from build123d import *

# Parameters (mm, degrees)
SKETCH1_W               = 50
SKETCH1_H               = 79
SKETCH1_R               = 1.7
SKETCH1_W_2             = 25.4
SKETCH1_H_2             = 47.625
BOSS_EXTRUDE1_DEPTH     = 5
SKETCH2_W               = 20
SKETCH2_H               = 5
BOSS_EXTRUDE2_DEPTH     = 50
FILLET1_R               = 10
CUT_EXTRUDE1_DEPTH      = 86.240835285
CUT_EXTRUDE1_DEPTH_BACK = 86.240835285
SKETCH3_R               = 2


with BuildPart() as part:
    # Sketch1 → Boss-Extrude1 (new body)
    with BuildSketch(Plane.XY):
        Rectangle(SKETCH1_W, SKETCH1_H)
        with Locations((-20, 0)):
            Circle(SKETCH1_R, mode=Mode.SUBTRACT)
        with Locations((20, 0)):
            Circle(SKETCH1_R, mode=Mode.SUBTRACT)
        Rectangle(SKETCH1_W_2, SKETCH1_H_2, mode=Mode.SUBTRACT)
    extrude(amount=BOSS_EXTRUDE1_DEPTH)

    # Sketch2 → Boss-Extrude2 (add)
    with BuildSketch(Plane.ZY.offset(25)):
        with Locations((-10, 37)):
            Rectangle(SKETCH2_W, SKETCH2_H)
        with Locations((-10, -37)):
            Rectangle(SKETCH2_W, SKETCH2_H)
    extrude(amount=-BOSS_EXTRUDE2_DEPTH)

    # Fillet1
    fillet1_edges = [part.edges().sort_by_distance(p)[0] for p in [
        (0, 34.5, 0),
        (0, -34.5, 0),
    ]]
    fillet(fillet1_edges, radius=FILLET1_R)

    # Sketch3 → Cut-Extrude1 (cut, two sides: drawn at the far end of the back side and taken through both)
    with BuildSketch(Plane(origin=(0, 39.5, 0), x_dir=(1, 0, 0), z_dir=(0, 1, 0)).offset(-CUT_EXTRUDE1_DEPTH_BACK)):
        with Locations((-17.5, 10)):
            Circle(SKETCH3_R)
        with Locations((-6, 10)):
            Circle(SKETCH3_R)
        with Locations(Location((6, 10, 0), (0, 0, 180))):
            Circle(SKETCH3_R)
        with Locations((17.5, 10)):
            Circle(SKETCH3_R)
    extrude(amount=CUT_EXTRUDE1_DEPTH + CUT_EXTRUDE1_DEPTH_BACK, mode=Mode.SUBTRACT)


solid = part.part
Here's how the part is built. I have some questions about the finished solid (model axes, mm). A direction names the side the tool comes from. Round coordinates to 2 decimals unless told otherwise and drop trailing zeros. Order: outer loops, then holes, each group sorted by start corner. A loop starts at its lowest first (then second) coordinate and runs counter-clockwise, first axis right, second up. Notation, with made-up numbers: M 43.25,20 L 51.25,20 A4 ccw 51.25,26 Z; hole C 21.25,45 d4. An arc over 180 degrees is marked long. Return JSON: item names as keys, results as strings. Group by question number.
1. Please list where these lines run through material, in increasing order: probe 1 along Y at (x, z) = (-14, -13); probe 2 along Y at (x, z) = (20, 4); probe 3 along Z at (x, y) = (-6, -35.95).
2. I'm going to push flat-ended pins straight in: pin 1 Ø12 at (x, y) = (-15.5, -24) entering from -Z; pin 2 Ø2.5 at (x, z) = (-17.5, -10) entering from -Y; pin 3 Ø1.5 at (x, y) = (13, -23) entering from -Z. Where does each tip first touch, or does it pass through?
3. If we section it at D-D on x = -17.5: List the corners of the cut face in (y, z) for me, then the cut area to 3 significant figures.
4. On a 3-axis mill with a long thin cutter (end or side, diameter ignored), from which of +Z, -Z, +X, -X, +Y, -Y can I reach the whole of each face in a straight line? I mean faces 3 (the face through (-18.974, 36.863, -11.352)), 4 (the face through (-12.7, 0, 2)), 5 (the face through (0.35, -31.65, -3.01)). Say none if no direction works.
5. If we section it at A-A on x = 6: List the corners of the cut face in (y, z) for me, then the cut area to 3 significant figures.
6. If we section it at B-B on z = -17: List the corners of the cut face in (x, y) for me, then the cut area to 3 significant figures.
7. If we mould it in two halves opening along Y, with no side actions, what happens to faces 1 (the face through (-6, 37, -12)), 2 (the face through (12.7, 0, 2))? For each: pulls with the +Y half, pulls with the -Y half, needs draft (parallel to the pull), parting line crosses it, or undercut.
8. If we section it at C-C on x = 0.5: List the corners of the cut face in (y, z) for me, then the cut area to 3 significant figures.
Reply:
{
 "1": {"probe 1": "-39.5 to -34.5, 34.5 to 39.5", "probe 2": "-39.5 to -1.7, 1.7 to 39.5", "probe 3": "-20 to -12, -8 to 5"},
 "2": {"pin 1": "z = -1.65", "pin 2": "through", "pin 3": "z = 0"},
 "3": {"outline": "M -39.5,-20 L -34.5,-20 L -34.5,-12 L -39.5,-12 Z; M -39.5,-8 L -34.3,-8 A10 cw -24.5,0 L 24.5,0 A10 cw 34.3,-8 L 39.5,-8 L 39.5,5 L -39.5,5 Z; M 34.5,-20 L 39.5,-20 L 39.5,-12 L 34.5,-12 Z", "area": "598 mm^2"},
 "4": {"face 3": "+Y, -Y", "face 4": "+Z, -Z", "face 5": "-Z, +X, -X"},
 "5": {"outline": "M -39.5,-20 L -34.5,-20 L -34.5,-12 L -39.5,-12 Z; M -39.5,-8 L -34.3,-8 A10 cw -24.5,0 L -23.81,0 L -23.81,5 L -39.5,5 Z; M 23.81,0 L 24.5,0 A10 cw 34.3,-8 L 39.5,-8 L 39.5,5 L 23.81,5 Z; M 34.5,-20 L 39.5,-20 L 39.5,-12 L 34.5,-12 Z", "area": "360 mm^2"},
 "6": {"outline": "M -25,-39.5 L 25,-39.5 L 25,-34.5 L -25,-34.5 Z; M -25,34.5 L 25,34.5 L 25,39.5 L -25,39.5 Z", "area": "500 mm^2"},
 "7": {"face 1": "needs draft", "face 2": "undercut"},
 "8": {"outline": "M -39.5,-20 L -34.5,-20 L -34.5,-10 A10 cw -24.5,0 L -23.81,0 L -23.81,5 L -39.5,5 Z; M 23.81,0 L 24.5,0 A10 cw 34.5,-10 L 34.5,-20 L 39.5,-20 L 39.5,5 L 23.81,5 Z", "area": "400 mm^2"}
}
